```python
from build123d import *

# Parameters (mm, degrees)
BOSS_EXTRUDE1_DEPTH             = 30
F_5_40_TAPPED_HOLE1_D           = 2.5781
F_5_40_TAPPED_HOLE1_DEPTH       = 15
F_5_40_TAPPED_HOLE1_CSINK_D     = 4.445
F_5_40_TAPPED_HOLE1_CSINK_ANGLE = 100
F_5_40_TAPPED_HOLE1_TIP         = 0.774539381
M4X0_7_TAPPED_HOLE1_D           = 3.3
M4X0_7_TAPPED_HOLE1_DEPTH       = 15
M4X0_7_TAPPED_HOLE1_TIP         = 0.991420021
SKETCH9_R                       = 3
CUT_EXTRUDE2_DEPTH              = 5
SKETCH10_R                      = 3
CUT_EXTRUDE3_DEPTH              = 5


with BuildPart() as part:
    # Sketch2 → Boss-Extrude1 (new body)
    with BuildSketch(Plane(origin=(0, 0, 0), x_dir=(1, 0, 0), z_dir=(0, 1, 0))):
        Polygon((3, 0), (1.5, 2.598076211), (-1.5, 2.598076211), (-3, 0), (-1.5, -2.598076211), (1.5, -2.598076211), align=None)
    extrude(amount=BOSS_EXTRUDE1_DEPTH)

    # #5-40 Tapped Hole1
    with Locations(Plane(origin=(0, 30, 0), x_dir=(1, 0, 0), z_dir=(0, 1, 0))):
        with Locations((0, 0)):
            CounterSinkHole(F_5_40_TAPPED_HOLE1_D / 2, F_5_40_TAPPED_HOLE1_CSINK_D / 2, depth=F_5_40_TAPPED_HOLE1_DEPTH, counter_sink_angle=F_5_40_TAPPED_HOLE1_CSINK_ANGLE)
            with Locations((0, 0, -(F_5_40_TAPPED_HOLE1_DEPTH + F_5_40_TAPPED_HOLE1_TIP / 2))):  # 118° drill point
                Cone(0, F_5_40_TAPPED_HOLE1_D / 2, F_5_40_TAPPED_HOLE1_TIP, mode=Mode.SUBTRACT)

    # M4x0.7 Tapped Hole1
    with Locations(Plane(origin=(-0.014516339, 0, -0.025143037), x_dir=(0, 0, -1), z_dir=(0, -1, 0))):
        with Locations((0, 0)):
            Hole(M4X0_7_TAPPED_HOLE1_D / 2, depth=M4X0_7_TAPPED_HOLE1_DEPTH)
            with Locations((0, 0, -(M4X0_7_TAPPED_HOLE1_DEPTH + M4X0_7_TAPPED_HOLE1_TIP / 2))):  # 118° drill point
                Cone(0, M4X0_7_TAPPED_HOLE1_D / 2, M4X0_7_TAPPED_HOLE1_TIP, mode=Mode.SUBTRACT)

    # Sketch9 → Cut-Extrude2 (cut)
    with BuildSketch(Plane(origin=(0, 30, 0), x_dir=(1, 0, 0), z_dir=(0, 1, 0))):
        Circle(SKETCH9_R)
    extrude(amount=-CUT_EXTRUDE2_DEPTH, mode=Mode.SUBTRACT)

    # Sketch10 → Cut-Extrude3 (cut)
    with BuildSketch(Plane.XZ):
        Circle(SKETCH10_R)
    extrude(amount=-CUT_EXTRUDE3_DEPTH, mode=Mode.SUBTRACT)


solid = part.part
```
Build history of the part. All positions in model axes, mm. Coordinates: 2 decimals unless noted, no trailing zeros. Write each loop counter-clockwise with the first axis right and the second up, starting at its lowest first coordinate (ties: lowest second). Pieces come first, ordered by that corner, then holes.
1. Drill centre lines: probe 1 along Z at (x, y) = (0, 17.75); probe 2 along X at (y, z) = (8.75, -1); probe 3 along X at (y, z) = (11, 1.2). Where is each one in solid material? Low to high.
Answer block:
probe 1: z = -2.6 to -1.29, 1.29 to 2.6
probe 2: x = -2.42 to -1.35, 1.32 to 2.42
probe 3: x = -2.31 to -1.12, 1.09 to 2.31
2. Drop a flat-ended pin along its axis: pin 1 (1.5 mm diameter, centred on y = 14.5, z = -0.5, fed in from +X). Give the stop position or say it passes through.
Answer block:
pin 1: stops at x = 3
3. Band-saw the part on B-B, the plane y = 12.25. Give the cut face in (x, z).
Answer block:
outline: (-3, 0) - (-1.5, -2.6) - (1.5, -2.6) - (3, 0) - (1.5, 2.6) - (-1.5, 2.6) - close; hole circle Ø3.3 at (-0.01, -0.03)
4. Band-saw the part on A-A, the plane y = 21.75. Give the cut face in (x, z).
Answer block:
outline: (-3, 0) - (-1.5, -2.6) - (1.5, -2.6) - (3, 0) - (1.5, 2.6) - (-1.5, 2.6) - close; hole circle Ø2.58 at (0, 0)
5. Pull direction Z, two halves, no side cores. Call faces 1 (the cylindrical face through (-0.69, 20.03, -1.09)), 2 (the cylindrical face through (1.1, 10.07, -1.24)), 3 (the flat face through (0, 15, 2.598)), 4 (the flat face through (2.26, 14.86, -1.28)): released by +Z, released by -Z, zero draft, split by the parting line, or undercut.
Answer block:
face 1: undercut
face 2: undercut
face 3: released by +Z
face 4: released by -Z
6. Band-saw the part on D-D, the plane x = -1.95. Give the cut face in (y, z), and give its area (3 significant figures).
Answer block:
outline: (5, -1.82) - (25, -1.82) - (25, 1.82) - (5, 1.82) - close
area: 72.7 mm2
7. Band-saw the part on C-C, the plane z = -1.9. Give the cut face in (x, y), and give its area (3 significant figures).
Answer block:
outline: (-1.9, 5) - (1.9, 5) - (1.9, 25) - (-1.9, 25) - close
area: 76.1 mm2
